```python
from build123d import *

# Parameters (mm, degrees)
F0_W     = 40.5096374452
F0_H     = 38.8049148023
F1_DEPTH = 138.684
F2_SIZE  = 5.08
F5_DEPTH = 26.416


with BuildPart() as f1:
    # F0 (on Front) → F1 (new body)
    with BuildSketch(Plane.XZ):
        with Locations((20.2548187226, 19.4024574012)):
            Rectangle(F0_W, F0_H)
    extrude(amount=F1_DEPTH)

    # F2
    f2_edges = [f1.edges().sort_by_distance(p)[0] for p in [
        (0, -69.342, 38.804915),
    ]]
    chamfer(f2_edges, length=F2_SIZE)

    # F4 (on face) → F5 (cut)
    with BuildSketch(Plane.XZ.offset(138.684)):
        Polygon((40.5096374452, 38.8049148023), (5.08, 38.8049148023), (0, 33.7249148023), (0, 0), (40.5096374452, 0), align=None)
        with BuildLine():
            Line((12.4323120505, 15.3702050447), (12.4323120505, 25.048552081))
            ThreePointArc((12.4323120505, 25.048552081), (18.7823120505, 31.398552081), (25.1323120505, 25.048552081))
            Line((25.1323120505, 25.048552081), (25.1323120505, 15.3702050447))
            ThreePointArc((25.1323120505, 15.3702050447), (18.7823120505, 9.0202050447), (12.4323120505, 15.3702050447))
        make_face(mode=Mode.SUBTRACT)
    extrude(amount=-F5_DEPTH, mode=Mode.SUBTRACT)


solid = f1.part
```
Work out the finished part from the listing and answer in its coordinate system (mm). A direction names the side the tool comes from. Give positions to 0.01 mm unless a question says otherwise; leave off trailing zeros. Loops run counter-clockwise (first coordinate to the right, second up) from the corner with the lowest first, then second, coordinate; pieces in that order, holes last. Notation, with made-up numbers: (81, -33.75) -> (119, -33.75) arc R23 cw to (119, 1.25) -> close; hole circle Ø2 at (-37, -18.75). An arc over 180 degrees is marked (long way). Write item = value, one per line. Start each with the question number.
(1) Find section C-C on y = -127. Give the vertices of the cut face in (x, z), and give its area (3 significant figures).
(2) Given pin 1 Ø5 at (y, z) = (-130.5, 18.5) entering from -X; pin 2 Ø6 at (x, z) = (31.5, 5) entering from -Y; pin 3 Ø5 at (y, z) = (-121.5, 21.5) entering from +X, each flat-ended and moving along its own axis, determine where each tip first touches the part or whether it passes through.
(3) Which of the six approach directions +Z, -Z, +X, -X, +Y, -Y give full straight-line access (tool end or side, diameter ignored) to faces 1 (the flat face through (40.51, -55, 19)), 2 (the flat face through (25.132, -126, 20)), 3 (the flat face through (12.432, -126, 20)), 4 (the cylindrical face through (18.643, -125.661, 31.397)), 5 (the cylindrical face through (18.92, -125.66, 9.02))?
(4) Find the intervals of material crossed by probe 1 along Y at (x, z) = (35.5, 8); probe 2 along X at (y, z) = (-116.5, 20.5); probe 3 along X at (y, z) = (-60, 37.5), in increasing order. Write a range as from..to.
(5) Find section D-D on z = 7. Give the vertices of the cut face in (x, y).
(6) Find section A-A on z = 18. Give the vertices of the cut face in (x, y), and give its area (3 significant figures).
(7) Find section B-B on x = 19. Give the vertices of the cut face in (y, z), and give its area (3 significant figures).
From the geometry:
q1.outline = (12.43, 15.37) arc R6.35 ccw to (25.13, 15.37) -> (25.13, 25.05) arc R6.35 ccw to (12.43, 25.05) -> close
q1.area = 250 mm^2
q2.pin_1 = 12.43
q2.pin_2 = -112.27
q2.pin_3 = 25.13
q3.face_1 = +Z, -Z, +X, +Y, -Y
q3.face_2 = +Z, -Z, +X, -Y
q3.face_3 = +Z, -Z, -X, -Y
q3.face_4 = +Z, -Y
q3.face_5 = -Z, -Y
q4.probe_1 = -112.27..0
q4.probe_2 = 12.43..25.13
q4.probe_3 = 3.78..40.51
q5.outline = (0, -112.27) -> (40.51, -112.27) -> (40.51, 0) -> (0, 0) -> close
q6.outline = (0, -112.27) -> (12.43, -112.27) -> (12.43, -138.68) -> (25.13, -138.68) -> (25.13, -112.27) -> (40.51, -112.27) -> (40.51, 0) -> (0, 0) -> close
q6.area = 4,880 mm^2
q7.outline = (-138.68, 9.02) -> (-112.27, 9.02) -> (-112.27, 0) -> (0, 0) -> (0, 38.8) -> (-112.27, 38.8) -> (-112.27, 31.39) -> (-138.68, 31.39) -> close
q7.area = 4,950 mm^2
